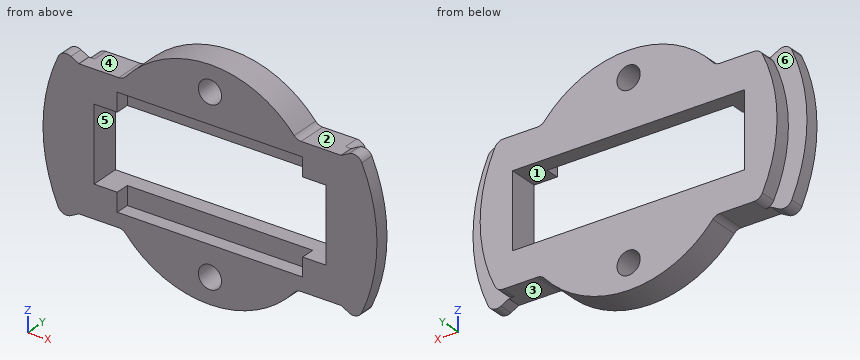
```python
from build123d import *

# Parameters (mm, degrees)
SKETCH1_W           = 40
SKETCH1_H           = 16
BOSS_EXTRUDE1_DEPTH = 6.4
SKETCH2_W           = 40
SKETCH2_H           = 4
CUT_EXTRUDE1_DEPTH  = 3
SKETCH3_W           = 5
SKETCH3_H           = 16
CUT_EXTRUDE2_DEPTH  = 7.4
BOSS_EXTRUDE2_DEPTH = 6.4
BOSS_EXTRUDE3_DEPTH = 3
FILLET1_R           = 2
SKETCH7_R           = 2.5
CUT_EXTRUDE3_DEPTH  = 7.4


with BuildPart() as part:
    # Sketch1 → Boss-Extrude1 (new body)
    with BuildSketch(Plane(origin=(0, 0, 0), x_dir=(1, 0, 0), z_dir=(0, 1, 0))):
        with BuildLine():
            Line((28.26658805, 15), (-28.26658805, 15))
            ThreePointArc((-28.26658805, 15), (-32, 0), (-28.26658805, -15))
            Line((-28.26658805, -15), (28.26658805, -15))
            ThreePointArc((28.26658805, -15), (32, 0), (28.26658805, 15))
        make_face()
        Rectangle(SKETCH1_W, SKETCH1_H, mode=Mode.SUBTRACT)
    extrude(amount=BOSS_EXTRUDE1_DEPTH)

    # Sketch2 → Cut-Extrude1 (cut)
    with BuildSketch(Plane.XZ):
        with Locations((0, 10)):
            Rectangle(SKETCH2_W, SKETCH2_H)
        with Locations((0, -10)):
            Rectangle(SKETCH2_W, SKETCH2_H)
    extrude(amount=-CUT_EXTRUDE1_DEPTH, mode=Mode.SUBTRACT)

    # Sketch3 → Cut-Extrude2 (cut, through all)
    with BuildSketch(Plane.XZ):
        with Locations((-22.5, 0)):
            Rectangle(SKETCH3_W, SKETCH3_H)
        with Locations((22.5, 0)):
            Rectangle(SKETCH3_W, SKETCH3_H)
    extrude(amount=-CUT_EXTRUDE2_DEPTH, mode=Mode.SUBTRACT)

    # Sketch5 → Boss-Extrude2 (add)
    with BuildSketch(Plane(origin=(0, 6.4, 0), x_dir=(1, 0, 0), z_dir=(0, 1, 0))):
        with BuildLine():
            Line((-18.734993995, -15), (18.734993995, -15))
            ThreePointArc((18.734993995, -15), (0, -24), (-18.734993995, -15))
        make_face()
        with BuildLine():
            Line((-18.734993995, 15), (18.734993995, 15))
            ThreePointArc((18.734993995, 15), (0, 24), (-18.734993995, 15))
        make_face()
    extrude(amount=-BOSS_EXTRUDE2_DEPTH)

    # Sketch6 → Boss-Extrude3 (add)
    with BuildSketch(Plane.XZ):
        with BuildLine():
            Line((-31.799911556, 16.875), (-28.26658805, 15))
            ThreePointArc((-28.26658805, 15), (-32, 0), (-28.26658805, -15))
            Line((-28.26658805, -15), (-31.799911556, -16.875))
            ThreePointArc((-31.799911556, -16.875), (-36, 0), (-31.799911556, 16.875))
        make_face()
        with BuildLine():
            ThreePointArc((31.799911556, 16.875), (36, 0), (31.799911556, -16.875))
            Line((31.799911556, -16.875), (28.26658805, -15))
            ThreePointArc((28.26658805, -15), (32, 0), (28.26658805, 15))
            Line((28.26658805, 15), (31.799911556, 16.875))
        make_face()
    extrude(amount=-BOSS_EXTRUDE3_DEPTH)

    # Fillet1
    fillet1_edges = [part.edges().sort_by_distance(p)[0] for p in [
        (-31.799911556, 1.5, 16.875),
        (-31.799911556, 1.5, -16.875),
        (31.799911556, 1.5, 16.875),
        (31.799911556, 1.5, -16.875),
        (28.26658805, 4.7, 15),
        (-28.26658805, 4.7, 15),
        (-28.26658805, 4.7, -15),
        (28.26658805, 4.7, -15),
        (-18.734993995, 3.2, 15),
        (18.734993995, 3.2, 15),
        (18.734993995, 3.2, -15),
        (-18.734993995, 3.2, -15),
    ]]
    fillet(fillet1_edges, radius=FILLET1_R)

    # Sketch7 → Cut-Extrude3 (cut, through all)
    with BuildSketch(Plane(origin=(0, 6.4, 0), x_dir=(1, 0, 0), z_dir=(0, 1, 0))):
        with Locations((0, 18.5)):
            Circle(SKETCH7_R)
        with Locations((0, -18.5)):
            Circle(SKETCH7_R)
    extrude(amount=-CUT_EXTRUDE3_DEPTH, mode=Mode.SUBTRACT)


solid = part.part
```
Could you check a few things on this model? Use its own coordinates, in mm. Face numbers are marked on the shaded views. A direction names the side the tool comes from. Coordinates: 2 decimals unless noted, no trailing zeros. Write each loop counter-clockwise with the first axis right and the second up, starting at its lowest first coordinate (ties: lowest second). Pieces come first, ordered by that corner, then holes. Notation, with made-up numbers: (39.5, -34.5) -> (46.5, -34.5) arc R29 ccw to (46.5, -1.5) -> close; hole circle Ø7 at (68.5, 78.25). An arc over 180 degrees is marked (long way). Return JSON: item names as keys, results as strings.
(1) I need wall thicknesses on L1, parallel to Z at x = -23, y = 1.5; L2, parallel to Z at x = -1, y = 2.75; L3, parallel to X at y = 2, z = 7. Which ranges of each line are inside material? Lowest first, please.
Numbers:
{"L1": "z = -15 to -8, 8 to 15", "L2": "z = -23.98 to -20.79, -16.21 to -12, 12 to 16.21, 20.79 to 23.98", "L3": "x = -35.31 to -25, 25 to 35.31"}
(2) Imagine slicing it at D-D, the plane z = 10. Please give me the cut outline in (x, y).
Numbers:
{"outline": "(-34.58, 0) -> (-20, 0) -> (-20, 3) -> (20, 3) -> (20, 0) -> (34.58, 0) -> (34.58, 3) -> (30.4, 3) -> (30.4, 6.4) -> (-30.4, 6.4) -> (-30.4, 3) -> (-34.58, 3) -> close"}
(3) Which directions (+Z, -Z, +X, -X, +Y, -Y) give clear straight access to the entire face, cutting with the end or side of a thin tool? Please do the marked faces 4, 5 and 6.
Numbers:
{"face 4": "+Z, +Y, -Y", "face 5": "+Y, -Y", "face 6": "-X, +Y"}
(4) Imagine slicing it at A-A, the plane x = 0. Please give me the cut outline in (y, z), then the cut area to 3 significant figures.
Numbers:
{"outline": "(0, -24) -> (6.4, -24) -> (6.4, -21) -> (0, -21) -> close; (0, -16) -> (6.4, -16) -> (6.4, -8) -> (3, -8) -> (3, -12) -> (0, -12) -> close; (0, 12) -> (3, 12) -> (3, 8) -> (6.4, 8) -> (6.4, 16) -> (0, 16) -> close; (0, 21) -> (6.4, 21) -> (6.4, 24) -> (0, 24) -> close", "area": "117 mm2"}
(5) Imagine slicing it at C-C, the plane z = -18.5. Please give me the cut outline in (x, y), then the cut area to 3 significant figures.
Numbers:
{"outline": "(-15.29, 0) -> (-2.5, 0) -> (-2.5, 6.4) -> (-15.29, 6.4) -> close; (2.5, 0) -> (15.29, 0) -> (15.29, 6.4) -> (2.5, 6.4) -> close", "area": "164 mm2"}
(6) We'd pull the mould along Z, two halves only. Please class the marked faces 1, 2 and 3: +Z half, -Z half, draft (parallel to the pull), parting line (faces both ways), or undercut.
Numbers:
{"face 1": "undercut", "face 2": "+Z half", "face 3": "-Z half"}
(7) Imagine slicing it at B-B, the plane y = 1. Count the separate pieces of the cut face and the enclosed holes in it, then the cut area to 3 significant figures.
Numbers:
{"separate pieces": "1", "enclosed holes": "3", "area": "1,420 mm2"}
(8) I'm going to push flat-ended pins straight in: pin 1 (1.5 mm diameter, centred on x = 18, y = 1, fed in from -Z); pin 2 (4 mm diameter, centred on x = 12.5, z = -8.5, fed in from -Y); pin 3 (2 mm diameter, centred on y = 3.5, z = -0.5, fed in from -X). Where does each tip first touch, or does it pass through?
Numbers:
{"pin 1": "stops at z = -16.69", "pin 2": "stops at y = 3", "pin 3": "stops at x = -36"}
